Autodesk Inventor part; units mm, degrees
ref_plane "YZ Plane" through (0, 0, 0) normal (1, 0, 0) x (0, 1, 0)
ref_plane "XZ Plane" through (0, 0, 0) normal (0, 1, 0) x (-1, 0, 0)
ref_plane "XY Plane" through (0, 0, 0) normal (0, 0, 1) x (1, 0, 0)
sketch "Sketch1" plane through (0, 0, 0) normal (0, 0, 1) x (1, 0, 0)
  line L0 (0, 52.8) -> (0, -8.8) construction
  line L1 (-18, 0) -> (3, 0) construction
  line L2 (-15, 0) -> (0, 0)
  line L3 (-15, 0) -> (-15, 25)
  line L4 (-15, 25) -> (-8, 44)
  line L5 (-8, 44) -> (0, 44)
  line L6 (0, 44) -> (0, 0)
  line L7 (-15, 0) -> (-14, 0)
  line L8 (-14, 0) -> (-14, 4.5)
  line L9 (-14, 4.5) -> (-15, 4.5)
  line L10 (-15, 4.5) -> (-15, 0)
  dimension "d0" = 15
  dimension "d1" = 44
  dimension "d2" = 8
  dimension "d3" = 25
  dimension "d31" = 1
  dimension "d32" = 4.5
revolve "Revolution1" add sketch "Sketch1" angle 360 about axis through (0, 0, 0) along (0, -1, 0)
revolve "Revolution4" cut sketch "Sketch1" angle 360 about axis through (0, 0, 0) along (0, -1, 0) contours L3 L9 L8 L2
sketch "Sketch2" plane through (0, 0, 0) normal (0, 0, 1) x (1, 0, 0)
  line L0 (-8, 44) -> (-15, 25)
  line L1 (-8, 44) -> (8, 44)
  line L2 (8, 44) -> (15, 25)
  line L3 (0, 44) -> (0, 20)
  line L4 (0, 20) -> (-12, 20)
  line L5 (-5, 44) -> (-12, 20)
  line L6 (0, 15.2) -> (0, 48.8)
  dimension "d10" = 12
  dimension "d11" = 3
  dimension "d12" = 24
revolve "Revolution2" cut sketch "Sketch2" angle 360 about axis through (0, -10, 0) along (0, 1, 0)
sketch "Sketch3" plane through (0, 0, 0) normal (0, -1, 0) x (1, 0, 0)
  circle A0 centre (0, 0) radius 15
hole "Hole1" at (0, 0, 0) direction (0, 1, 0) diameter 11.835 depth 20
sketch "Sketch4" plane through (0, 0, 0) normal (0, 0, 1) x (1, 0, 0)
  line L0 (-15, 0) -> (15, 0)
  line L1 (-15, 25) -> (15, 25)
  line L2 (-15, 25) -> (-15, 0)
  line L3 (-15, 25) -> (-16, 25)
  line L4 (-16, 25) -> (-16, 18)
  line L5 (-16, 18) -> (-15, 18)
  line L6 (-15, 18) -> (-15, 25)
  line L7 (-15, 11.5) -> (-16, 11.5)
  line L8 (-16, 11.5) -> (-16, 4.5)
  line L9 (-16, 4.5) -> (-15, 4.5)
  line L10 (-15, 4.5) -> (-15, 11.5)
  line L11 (0, -5) -> (0, 30)
  line L12 (15, 4.5) -> (-15, 4.5)
  point P0 (-15.5, 11.5)
  point P1 (-15.5, 18)
  point P2 (-15, 8)
  point P3 (-15, 18)
  dimension "d24" = 1
  dimension "d28" = 7
  dimension "d29" = 7
revolve "Revolution3" add sketch "Sketch4" angle 360 about axis through (0, -10, 0) along (0, 1, 0) contours L9 L8 L7 L2 | L5 L4 L3 L2
properties part number "B3OFT4_HF2_kezifuro_Tokmany" material "Stainless Steel"
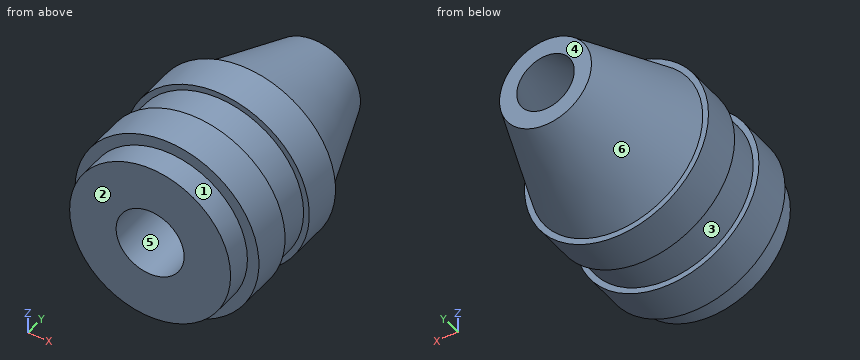
Can you work these out from the model? Positions are in its coordinate system, mm. Face numbers are marked on the shaded views. A direction names the side the tool comes from. Coordinates: 2 decimals unless noted, no trailing zeros. Write each loop counter-clockwise with the first axis right and the second up, starting at its lowest first coordinate (ties: lowest second). Pieces come first, ordered by that corner, then holes. Notation, with made-up numbers: M 9.25,55.25 L 14.25,55.25 A24 cw 14.25,70.25 Z; hole C 21.25,64.5 d2. An arc over 180 degrees is marked long. Write item = value, one per line. Start each with the question number.
Q1. I'm going to push flat-ended pins straight in: pin 1 (1.5 mm diameter, centred on x = -7, y = 39, fed in from -Z); pin 2 (6 mm diameter, centred on y = 27.5, z = 4, fed in from -X); pin 3 (6 mm diameter, centred on x = -9, y = 26, fed in from +Z). Where does each tip first touch, or does it pass through?
Q2. If we section it at C-C, the plane y = 7.5: Write out the boundary of the cut face in (x, z) (1 decimal), then the cut area to 3 significant figures.
Q3. If we section it at B-B, the plane y = 12.5: Write out the boundary of the cut face in (x, z) (1 decimal).
Q4. Thinking about a two-plate mould opening in Z: for the marked faces 4, 5 and 6, which applies, released by +Z, released by -Z, zero draft, split by the parting line, or undercut?
Q5. On a 3-axis mill with a long thin cutter (end or side, diameter ignored), from which of +Z, -Z, +X, -X, +Y, -Y can I reach the whole of each face in a straight line? I mean the marked faces 1, 2 and 3. Say none if no direction works.
Q6. If I drill on L1, parallel to Z at x = 0, y = 12; L2, parallel to Z at x = 0, y = 11; L3, parallel to X at y = 28.5, z = -0.5, over which ranges is the centre line in solid material (lowest first)? Write a range as [from, to].
Q7. If we section it at A-A, the plane x = 0: Write out the boundary of the cut face in (y, z), then the cut area to 3 significant figures.
Check sheet entries:
q1.pin_1 = -7.7
q1.pin_2 = -15.83
q1.pin_3 = 14.76
q2.outline = C 0,0 d32; hole C 0,0 d11.8
q2.area = 694 mm²
q3.outline = C 0,0 d30; hole C 0,0 d11.8
q4.face_4 = zero draft
q4.face_5 = undercut
q4.face_6 = split by the parting line
q5.face_1 = -Y
q5.face_2 = +Z, -Z, +X, -X, -Y
q5.face_3 = none
q6.L1 = [-15, -5.92], [5.92, 15]
q6.L2 = [-16, -5.92], [5.92, 16]
q6.L3 = [-13.7, -9.51], [9.51, 13.7]
q7.outline = M 0,-14 L 4.5,-14 L 4.5,-16 L 11.5,-16 L 11.5,-15 L 18,-15 L 18,-16 L 25,-16 L 25,-15 L 44,-8 L 44,-5 L 20,-12 L 20,-5.92 L 0,-5.92 Z; M 0,5.92 L 20,5.92 L 20,12 L 44,5 L 44,8 L 25,15 L 25,16 L 18,16 L 18,15 L 11.5,15 L 11.5,16 L 4.5,16 L 4.5,14 L 0,14 Z
q7.area = 561 mm²
